```python
from build123d import *

# Parameters (mm, degrees)
F0_R     = 9.525
F1_DEPTH = 16.7005
F3_DEPTH = 4.6228
F4_R     = 9.525
F5_DEPTH = 8.2804


with BuildPart() as f1:
    # F0 (on Top) → F1 (new body)
    with BuildSketch(Plane.XY):
        Circle(F0_R)
    extrude(amount=F1_DEPTH)

    # F2 (on face) → F3 (cut)
    with BuildSketch(Plane.XY.offset(16.7005)):
        with BuildLine():
            ThreePointArc((2.3495, 9.230681), (0, 9.525), (-2.3495, 9.230681))
            Line((-2.3495, 9.230681), (-2.3495, -9.230681))
            ThreePointArc((-2.3495, -9.230681), (0, -9.525), (2.3495, -9.230681))
            Line((2.3495, -9.230681), (2.3495, 9.230681))
        make_face()
    extrude(amount=-F3_DEPTH, mode=Mode.SUBTRACT)

    # F4 (on face) → F5 (cut)
    with BuildSketch(Plane(origin=(0, 0, 0), x_dir=(1, 0, 0), z_dir=(0, 0, -1))):
        Circle(F4_R)
        with BuildLine():
            ThreePointArc((-6.646603, -3.175), (-7.366, 0), (-6.646603, 3.175))
            Line((-6.646603, 3.175), (6.646603, 3.175))
            ThreePointArc((6.646603, 3.175), (7.366, 0), (6.646603, -3.175))
            Line((6.646603, -3.175), (-6.646603, -3.175))
        make_face(mode=Mode.SUBTRACT)
    extrude(amount=-F5_DEPTH, mode=Mode.SUBTRACT)


solid = f1.part
```
Can you work these out from the model? Positions are in its coordinate system, mm. A direction names the side the tool comes from. Round coordinates to 2 decimals unless told otherwise and drop trailing zeros. Loops run counter-clockwise (first coordinate to the right, second up) from the corner with the lowest first, then second, coordinate; pieces in that order, holes last. Notation, with made-up numbers: M -34,38 L -24,38 A33 ccw -24,69 Z; hole C -14,41 d3. An arc over 180 degrees is marked long. Write item = value, one per line. Start each with the question number.
(1) Suppose I cut it at B-B on y = 0. Write out the boundary of the cut face in (x, z) (1 decimal).
(2) If we mould it in two halves opening along X, with no side actions, what happens to faces 1 (the face through (2.35, 0, 14)), 2 (the face through (7.366, -0.046, 4.082)), 3 (the face through (-7.366, 0.046, 4.082))? For each: released by +X, released by -X, zero draft, split by the parting line, or undercut.
(3) Which directions (+Z, -Z, +X, -X, +Y, -Y) give clear straight access to the entire face, cutting with the end or side of a thin tool? Please do faces 4 (the face through (0, 0, 12.078)), 5 (the face through (0, 3.175, 4)), 6 (the face through (0, -3.175, 4)).
(4) I'm going to push flat-ended pins straight in: P1, Ø1.4, axis at y = 1.5, z = 15, coming from the +X side; P2, Ø2, axis at x = 5.5, z = 15, coming from the +Y side (3 decimals); P3, Ø9, axis at x = -1, z = 4, coming from the -Y side (3 decimals); P4, Ø1, axis at x = 1, y = -4, coming from the -Z side. Where does each tip first touch, or does it pass through?
(5) Suppose I cut it at A-A on x = 0. Write out the boundary of the cut face in (y, z) (3 decimals).
(6) I need wall thicknesses on line 1 along Z through (x, y) = (8, -4.75); line 2 along Y through (x, z) = (2.5, 1.25) (3 decimals); line 3 along Z through (x, y) = (-1, 5.5). Which ranges of each line are inside material? Lowest first, please.
(7) Suppose I cut it at D-D on z = 1. Write out the boundary of the cut face in (x, y) (3 decimals), plus the area to 3 significant figures.
Answer block:
q1.outline = M -9.5,8.3 L -7.4,8.3 L -7.4,0 L 7.4,0 L 7.4,8.3 L 9.5,8.3 L 9.5,16.7 L 2.3,16.7 L 2.3,12.1 L -2.3,12.1 L -2.3,16.7 L -9.5,16.7 Z
q2.face_1 = undercut
q2.face_2 = released by +X
q2.face_3 = released by -X
q3.face_4 = +Z, +Y, -Y
q3.face_5 = -Z, +X, -X, +Y
q3.face_6 = -Z, +X, -X, -Y
q4.P1 = 9.49
q4.P2 = 8.395
q4.P3 = -9.525
q4.P4 = 8.28
q5.outline = M -9.525,8.28 L -3.175,8.28 L -3.175,0 L 3.175,0 L 3.175,8.28 L 9.525,8.28 L 9.525,12.078 L -9.525,12.078 Z
q6.line_1 = 8.28 to 16.7
q6.line_2 = -3.175 to 3.175
q6.line_3 = 8.28 to 12.08
q7.outline = M -6.647,-3.175 L 6.647,-3.175 A7.366 ccw 6.647,3.175 L -6.647,3.175 A7.366 ccw Z
q7.area = 90.6 mm²
